Input: part model. Units: mm. Frame: model coordinates. Coordinates: 2 decimals unless noted, no trailing zeros. Loops run counter-clockwise (first coordinate to the right, second up) from the corner with the lowest first, then second, coordinate; pieces in that order, holes last.
Item 1: Ray query, line 1 along X through (y, z) = (-55.5, 0.25) (3 decimals); line 2 along X through (y, z) = (47.5, 1.85); line 3 along Y through (x, z) = (75, 1.1). Return the intervals inside material, ascending.
Item 2: Contact query for flat-ended pins moving along their axis: P1, Ø5, axis at x = -38.1, y = 63.5, coming from the +Z side (3 decimals); P2, Ø1.5, axis at y = 11.5, z = 2.5, coming from the +X side; P3, Ø1, axis at x = -97, z = 1, coming from the -Y side; P4, Ø1.6, axis at y = -60.5, z = 2.5, coming from the -X side (3 decimals). Output: stop coordinate, or through.
Item 3: Section D-D on x = -32. Return loops of the section in (y, z) (3 decimals), and give its area (3 significant figures).
Item 4: Section B-B on z = 1.05. Give the number of separate pieces and of enclosed holes in the cut face, and give its area (3 significant figures).
Item 5: Section C-C on y = -53. Return loops of the section in (x, z) (3 decimals), and give its area (3 significant figures).
Item 6: Section A-A on x = 63.5. Return loops of the section in (y, z) (3 decimals).
Autodesk Inventor part; units mm, degrees
ref_plane "YZ Plane" through (0, 0, 0) normal (1, 0, 0) x (0, 1, 0)
ref_plane "XZ Plane" through (0, 0, 0) normal (0, 1, 0) x (-1, 0, 0)
ref_plane "XY Plane" through (0, 0, 0) normal (0, 0, 1) x (1, 0, 0)
sketch "Sketch1" plane through (0, 0, 0) normal (0, 0, 1) x (1, 0, 0)
  line L0 (-101.6, -76.2) -> (101.6, -76.2)
  line L1 (101.6, -76.2) -> (101.6, 76.2)
  line L2 (101.6, 76.2) -> (-101.6, 76.2)
  line L3 (-101.6, 76.2) -> (-101.6, -76.2)
  line L4 (-101.6, -76.2) -> (101.6, 76.2) construction
  line L5 (101.6, -76.2) -> (-101.6, 76.2) construction
  point P0 (0, 0)
  dimension "d0" = 152.4
  dimension "d1" = 203.2
extrude "Extrusion1" add sketch "Sketch1" along normal blind 3.175
sketch "Sketch2" plane through (0, 0, 0) normal (0, 0, -1) x (-1, 0, 0)
  circle A0 centre (-37.1038, -82.4738) radius 101.092
  circle A1 centre (-37.1038, -82.4738) radius 107.442
  line L0 (-101.6, -76.2) -> (-101.6, 76.2)
  line L1 (-101.6, 3.4565) -> (-101.6, -76.2)
  line L2 (-101.6, -76.2) -> (70.1549, -76.2)
  line L3 (101.6, -76.2) -> (-101.6, -76.2)
  point P0 (0, 0)
  dimension "d4" = 214.884
extrude "Extrusion2" cut sketch "Sketch2" against normal blind 25.4 contours L2 L0 A0 | A0 L0 A1 L2 picked at (8.0579, -71.6086) picked at (67.4292, -71.4153)
fillet "Fillet1" radius 12.7 5 edges at (101.6, 76.2, 1.5875) (-101.6, 76.2, 1.5875) (-101.6, -76.2, 1.5875) (-70.1549, -76.2, 1.5875) (101.6, 3.4565, 1.5875)
sketch "Sketch3" plane through (0, 0, 0) normal (0, 0, -1) x (-1, 0, 0)
  line L0 (76.2027, 73.1012) -> (-660.4, 73.1012)
  line L1 (-660.4, 53.8988) -> (76.2027, 53.8988)
  circle A0 centre (-647.7, 63.5) radius 2.0701
  circle A1 centre (-622.3, 63.5) radius 2.0701
  circle A2 centre (-596.9, 63.5) radius 2.0701
  circle A3 centre (-571.5, 63.5) radius 2.0701
  circle A4 centre (-546.1, 63.5) radius 2.0701
  circle A5 centre (-520.7, 63.5) radius 2.0701
  circle A6 centre (-495.3, 63.5) radius 2.0701
  circle A7 centre (-469.9, 63.5) radius 2.0701
  circle A8 centre (-444.5, 63.5) radius 2.0701
  circle A9 centre (-419.1, 63.5) radius 2.0701
  circle A10 centre (-393.7, 63.5) radius 2.0701
  circle A11 centre (-368.3, 63.5) radius 2.0701
  circle A12 centre (-342.9, 63.5) radius 2.0701
  circle A13 centre (-317.5, 63.5) radius 2.0701
  circle A14 centre (-292.1, 63.5) radius 2.0701
  circle A15 centre (-266.7, 63.5) radius 2.0701
  circle A16 centre (-241.3, 63.5) radius 2.0701
  circle A17 centre (-215.9, 63.5) radius 2.0701
  circle A18 centre (-190.5, 63.5) radius 2.0701
  circle A19 centre (-165.1, 63.5) radius 2.0701
  circle A20 centre (-139.7, 63.5) radius 2.0701
  circle A21 centre (-114.3, 63.5) radius 2.0701
  circle A22 centre (-88.9, 63.5) radius 2.0701
  circle A23 centre (-63.5, 63.5) radius 2.0701
  circle A24 centre (-38.1, 63.5) radius 2.0701
  circle A25 centre (-12.7, 63.5) radius 2.0701
  circle A26 centre (12.7, 63.5) radius 2.0701
  circle A27 centre (38.1, 63.5) radius 2.0701
  circle A28 centre (63.5, 63.5) radius 2.0701
  line L2 (97.2058, -44.2468) -> (78.359, -44.2468)
  line L3 (78.359, -44.2468) -> (76.2, -42.0878)
  line L4 (76.2, 16.8402) -> (76.2, -42.0878)
  line L5 (76.2, 16.8402) -> (78.359, 18.9992)
  line L6 (97.2058, 18.9992) -> (78.359, 18.9992)
  line L7 (97.2058, -44.2468) -> (97.2058, 18.9992)
  circle A29 centre (88.9, 12.7762) radius 2.0701
  circle A30 centre (88.9, 0.0762) radius 2.0701
  circle A31 centre (88.9, -12.6238) radius 2.0701
  circle A32 centre (88.9, -25.3238) radius 2.0701
  circle A33 centre (88.9, -38.0238) radius 2.0701
  line L8 (76.2027, 73.1012) -> (76.2027, 53.8988)
  line L9 (-660.4, 53.8988) -> (-660.4, 73.1012)
  point P0 (0, 0)
  point P1 (88.9, 25.4762)
  point P2 (88.9, 38.1762)
  dimension "d17" = 12.7
hole "Hole1" at (88.9, 63.5, 0) at (63.5, 63.5, 0) at (38.1, 63.5, 0) at (12.7, 63.5, 0) at (-12.7, 63.5, 0) at (-38.1, 63.5, 0) at (-63.5, 63.5, 0) at (-88.9, 12.7762, 0) at (-88.9, 0.0762, 0) at (-88.9, -12.6238, 0) at (-88.9, -25.3238, 0) at (-88.9, -38.0238, 0) at (-88.9, 25.4762, 0) at (-88.9, 38.1762, 0) direction (0, 0, 1) diameter 4.1402 end through all
sketch "Sketch4" plane through (0, 0, 0) normal (0, 0, -1) x (-1, 0, 0)
  line L0 (-88.9, 76.2) -> (88.9, 76.2)
  line L1 (-25.4, 76.2) -> (25.4, 76.2)
  line L2 (25.4, 76.2) -> (25.4, 44.45)
  line L3 (25.4, 44.45) -> (-25.4, 44.45)
  line L4 (-25.4, 44.45) -> (-25.4, 76.2)
  line L5 (-101.6, 25.9294) -> (-101.6, 63.5)
  point P0 (0, 0)
  dimension "d23" = 31.75
  dimension "d24" = 50.8
  dimension "d25" = 76.2
extrude "Extrusion3" cut sketch "Sketch4" against normal through all
fillet "Fillet2" radius 12.7 4 edges at (25.4, 76.2, 1.5875) (25.4, 44.45, 1.5875) (-25.4, 44.45, 1.5875) (-25.4, 76.2, 1.5875)
sketch "Sketch5" plane through (0, 0, 3.175) normal (0, 0, 1) x (1, 0, 0)
  line L0 (-76.2, -76.1238) -> (-76.2, -25.4)
  line L1 (-76.2, -25.4) -> (-88.8238, -25.4)
  line L2 (-88.8238, -25.4) -> (-88.9, -25.4762)
  line L3 (-88.9, -25.4762) -> (-88.9762, -25.4)
  line L4 (-88.9762, -25.4) -> (-101.6, -25.4)
  line L5 (-101.6, -25.4) -> (-101.6, -76.1238)
  line L6 (-76.2, -76.1238) -> (-101.6, -76.1238)
  line L7 (-78.74, -27.94) -> (-78.74, -73.66)
  line L8 (-78.74, -73.66) -> (-99.06, -73.66)
  line L9 (-99.06, -73.66) -> (-99.06, -27.94)
  line L10 (-99.06, -27.94) -> (-78.74, -27.94)
  line L11 (-92.71, -31.75) -> (-92.71, -34.925)
  line L12 (-92.71, -31.75) -> (-99.06, -31.75)
  line L13 (-92.71, -66.675) -> (-92.71, -34.925)
  line L14 (-92.71, -66.675) -> (-92.71, -69.85)
  line L15 (-101.6, -25.4) -> (-92.075, -25.4)
  line L16 (-92.075, -25.4) -> (-92.075, -76.1238)
  line L17 (-92.075, -76.1238) -> (-101.6, -76.1238)
  line L18 (-101.6, -76.1238) -> (-101.6, -25.4)
  circle A0 centre (-88.9, -38.0238) radius 2.0701
  point P0 (0, 0)
  point P1 (-88.9, -76.2)
  dimension "d35" = 0.635
extrude "Extrusion4" cut sketch "Sketch5" against normal through all contours L6 L5 L4 L16 L10 L9 L8 | L8 L9 L10 L16
fillet "Fillet3" radius 3.175 3 edges at (-101.6, -25.4, 1.5875) (-92.075, -25.4, 1.5875) (-92.075, -75.7967, 1.5875)
properties part number "C13R1_TK_UpperFrameSupportWheel" material "Polycarbonate, Clear"
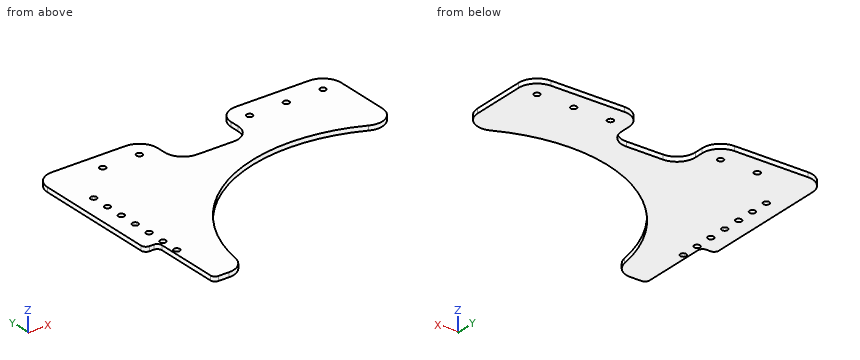
Results found:
1. line 1: x = -92.075 to -66.897
1. line 2: x = -101.6 to -20.96, 20.96 to 101.6
1. line 3: y = 18.06 to 76.2
2. P1: stops at z = 3.175
2. P2: stops at x = -13.6
2. P3: stops at y = -25.4
2. P4: stops at x = -92.075
3. outline: (-0.203, 0) - (74.639, 0) - (74.639, 3.175) - (-0.203, 3.175) - close
3. area: 238 mm2
4. separate pieces: 1
4. enclosed holes: 12
4. area: 14,000 mm2
5. outline: (-92.075, 0) - (-66.216, 0) - (-66.216, 3.175) - (-92.075, 3.175) - close
5. area: 82.1 mm2
6. outline: (21.675, 0) - (61.43, 0) - (61.43, 3.175) - (21.675, 3.175) - close; (65.57, 0) - (76.2, 0) - (76.2, 3.175) - (65.57, 3.175) - close
